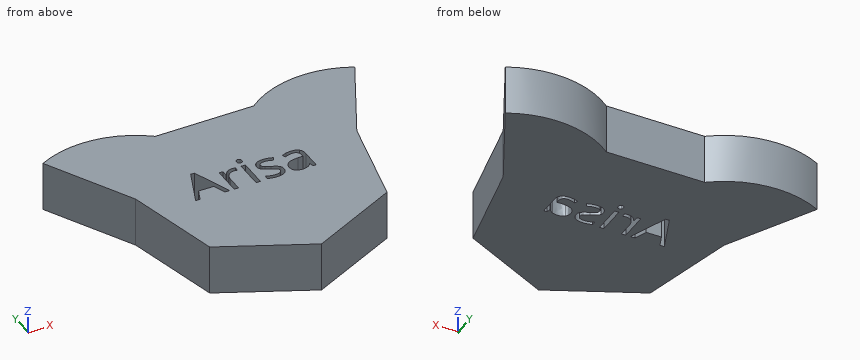
```python
from build123d import *

# Parameters (mm, degrees)
F0_W       = 2.2281454939
F0_H       = 14.7040429991
F1_DEPTH   = 25.4
F1_FACE_W  = 50.8
F1_FACE_H  = 25.4
F2_ANGLE   = 66
F1_FACE1_W = 50.8
F1_FACE1_H = 25.4
F3_ANGLE   = 66


with BuildPart() as f1:
    # F0 (on Top) → F1 (new body)
    with BuildSketch(Plane.XY):
        Polygon((-26.2134087423, 52.3441413045), (-57.2680906174, 12.1415700729), (-45.1987322015, -37.2038510665), (0.9061934483, -58.5340135326), (46.3287369485, -35.7868699324), (56.8647965925, 13.9085166461), (24.5805045719, 53.130506508), align=None)
        Polygon((-16.3552618695, -1.5368833827), (-18.7164950518, -1.5368833827), (-21.1592981077, 4.7010653699), (-29.0200580293, 4.7010653699), (-31.4328090265, -1.5368833827), (-33.742524394, -1.5368833827), (-25.9890932534, 18.1600945092), (-24.0700546489, 18.1600945092), align=None, mode=Mode.SUBTRACT)
        with BuildLine():
            add(Edge.make_bspline(
                [(-9.8210856812, 12.6584211944), (-8.6662279975, 13.4376281445), (-7.283833298, 13.4376281445)],
                knots=[0, 0, 0, 1, 1, 1], degree=2))
            add(Edge.make_bspline(
                [(-7.283833298, 13.4376281445), (-6.3049948152, 13.4376281445), (-5.5279344406, 13.2744883974)],
                knots=[0, 0, 0, 1, 1, 1], degree=2))
            Line((-5.5279344406, 13.2744883974), (-5.8370413299, 11.2094826507))
            add(Edge.make_bspline(
                [(-5.8370413299, 11.2094826507), (-6.747189393, 11.411260759), (-7.4469730452, 11.411260759)],
                knots=[0, 0, 0, 1, 1, 1], degree=2))
            add(Edge.make_bspline(
                [(-7.4469730452, 11.411260759), (-9.2329239613, 11.411260759), (-10.4994035773, 9.9623222153)],
                knots=[0, 0, 0, 1, 1, 1], degree=2))
            add(Edge.make_bspline(
                [(-10.4994035773, 9.9623222153), (-11.7658831932, 8.5133836715), (-11.7658831932, 6.3539285975)],
                knots=[0, 0, 0, 1, 1, 1], degree=2))
            Line((-11.7658831932, 6.3539285975), (-11.7658831932, -1.5368833827))
            Line((-11.7658831932, -1.5368833827), (-13.9940286871, -1.5368833827))
            Line((-13.9940286871, -1.5368833827), (-13.9940286871, 13.1671596164))
            Line((-13.9940286871, 13.1671596164), (-12.1565599561, 13.1671596164))
            Line((-12.1565599561, 13.1671596164), (-11.8989708817, 10.4453017298))
            Line((-11.8989708817, 10.4453017298), (-11.7916421007, 10.4453017298))
            add(Edge.make_bspline(
                [(-11.7916421007, 10.4453017298), (-10.975943365, 11.8792142442), (-9.8210856812, 12.6584211944)],
                knots=[0, 0, 0, 1, 1, 1], degree=2))
        make_face(mode=Mode.SUBTRACT)
        with Locations((-1.6619517484, 5.8151381168)):
            Rectangle(F0_W, F0_H, mode=Mode.SUBTRACT)
        with BuildLine():
            add(Edge.make_bspline(
                [(-2.5892724164, 16.0306914939), (-2.96492315, 16.3999025006), (-2.96492315, 17.1512039677)],
                knots=[0, 0, 0, 1, 1, 1], degree=2))
            add(Edge.make_bspline(
                [(-2.96492315, 17.1512039677), (-2.96492315, 17.9153848885), (-2.5892724164, 18.2717164415)],
                knots=[0, 0, 0, 1, 1, 1], degree=2))
            add(Edge.make_bspline(
                [(-2.5892724164, 18.2717164415), (-2.2136216829, 18.6280479944), (-1.6469257191, 18.6280479944)],
                knots=[0, 0, 0, 1, 1, 1], degree=2))
            add(Edge.make_bspline(
                [(-1.6469257191, 18.6280479944), (-1.110281814, 18.6280479944), (-0.7217516267, 18.2652767146)],
                knots=[0, 0, 0, 1, 1, 1], degree=2))
            add(Edge.make_bspline(
                [(-0.7217516267, 18.2652767146), (-0.3332214395, 17.9025054348), (-0.3332214395, 17.1512039677)],
                knots=[0, 0, 0, 1, 1, 1], degree=2))
            add(Edge.make_bspline(
                [(-0.3332214395, 17.1512039677), (-0.3332214395, 16.3999025006), (-0.7217516267, 16.0306914939)],
                knots=[0, 0, 0, 1, 1, 1], degree=2))
            add(Edge.make_bspline(
                [(-0.7217516267, 16.0306914939), (-1.110281814, 15.6614804872), (-1.6469257191, 15.6614804872)],
                knots=[0, 0, 0, 1, 1, 1], degree=2))
            add(Edge.make_bspline(
                [(-1.6469257191, 15.6614804872), (-2.2136216829, 15.6614804872), (-2.5892724164, 16.0306914939)],
                knots=[0, 0, 0, 1, 1, 1], degree=2))
        make_face(mode=Mode.SUBTRACT)
        with BuildLine():
            add(Edge.make_bspline(
                [(12.7394240882, 4.9028434782), (13.6581584537, 3.936884449), (13.6581584537, 2.472919876)],
                knots=[0, 0, 0, 1, 1, 1], degree=2))
            add(Edge.make_bspline(
                [(13.6581584537, 2.472919876), (13.6581584537, 0.420793583), (12.129796612, -0.693279164)],
                knots=[0, 0, 0, 1, 1, 1], degree=2))
            add(Edge.make_bspline(
                [(12.129796612, -0.693279164), (10.6014347704, -1.8073519109), (7.8366453714, -1.8073519109)],
                knots=[0, 0, 0, 1, 1, 1], degree=2))
            add(Edge.make_bspline(
                [(7.8366453714, -1.8073519109), (4.9130093766, -1.8073519109), (3.2773187539, -0.8800312429)],
                knots=[0, 0, 0, 1, 1, 1], degree=2))
            Line((3.2773187539, -0.8800312429), (3.2773187539, 1.1849745038))
            add(Edge.make_bspline(
                [(3.2773187539, 1.1849745038), (4.3377271103, 0.6483305987), (5.5505423358, 0.341370285)],
                knots=[0, 0, 0, 1, 1, 1], degree=2))
            add(Edge.make_bspline(
                [(5.5505423358, 0.341370285), (6.7633575613, 0.0344099713), (7.8924563376, 0.0344099713)],
                knots=[0, 0, 0, 1, 1, 1], degree=2))
            add(Edge.make_bspline(
                [(7.8924563376, 0.0344099713), (9.6354757412, 0.0344099713), (10.5735292873, 0.590373057)],
                knots=[0, 0, 0, 1, 1, 1], degree=2))
            add(Edge.make_bspline(
                [(10.5735292873, 0.590373057), (11.5115828334, 1.1463361426), (11.5115828334, 2.2883143727)],
                knots=[0, 0, 0, 1, 1, 1], degree=2))
            add(Edge.make_bspline(
                [(11.5115828334, 2.2883143727), (11.5115828334, 3.1469446208), (10.7688676688, 3.7565720969)],
                knots=[0, 0, 0, 1, 1, 1], degree=2))
            add(Edge.make_bspline(
                [(10.7688676688, 3.7565720969), (10.0261525041, 4.3661995731), (7.8624042789, 5.1990709138)],
                knots=[0, 0, 0, 1, 1, 1], degree=2))
            add(Edge.make_bspline(
                [(7.8624042789, 5.1990709138), (5.8102779859, 5.9632518346), (4.9452080109, 6.5342409496)],
                knots=[0, 0, 0, 1, 1, 1], degree=2))
            add(Edge.make_bspline(
                [(4.9452080109, 6.5342409496), (4.0801380359, 7.1052300646), (3.6572626387, 7.8286260487)],
                knots=[0, 0, 0, 1, 1, 1], degree=2))
            add(Edge.make_bspline(
                [(3.6572626387, 7.8286260487), (3.2343872415, 8.5520220327), (3.2343872415, 9.556619423)],
                knots=[0, 0, 0, 1, 1, 1], degree=2))
            add(Edge.make_bspline(
                [(3.2343872415, 9.556619423), (3.2343872415, 11.3554497928), (4.6983518145, 12.3965389687)],
                knots=[0, 0, 0, 1, 1, 1], degree=2))
            add(Edge.make_bspline(
                [(4.6983518145, 12.3965389687), (6.1623163876, 13.4376281445), (8.7081550733, 13.4376281445)],
                knots=[0, 0, 0, 1, 1, 1], degree=2))
            add(Edge.make_bspline(
                [(8.7081550733, 13.4376281445), (11.0822677093, 13.4376281445), (13.3533447156, 12.4716691154)],
                knots=[0, 0, 0, 1, 1, 1], degree=2))
            Line((13.3533447156, 12.4716691154), (12.5591117361, 10.6599592919))
            add(Edge.make_bspline(
                [(12.5591117361, 10.6599592919), (10.3481388472, 11.5701073549), (8.5493084774, 11.5701073549)],
                knots=[0, 0, 0, 1, 1, 1], degree=2))
            add(Edge.make_bspline(
                [(8.5493084774, 11.5701073549), (6.9651356696, 11.5701073549), (6.160169812, 11.0742483866)],
                knots=[0, 0, 0, 1, 1, 1], degree=2))
            add(Edge.make_bspline(
                [(6.160169812, 11.0742483866), (5.3552039544, 10.5783894183), (5.3552039544, 9.7068797164)],
                knots=[0, 0, 0, 1, 1, 1], degree=2))
            add(Edge.make_bspline(
                [(5.3552039544, 9.7068797164), (5.3552039544, 9.1144248452), (5.6578711168, 8.7001357505)],
                knots=[0, 0, 0, 1, 1, 1], degree=2))
            add(Edge.make_bspline(
                [(5.6578711168, 8.7001357505), (5.9605382793, 8.2858466558), (6.6302698728, 7.9101959222)],
                knots=[0, 0, 0, 1, 1, 1], degree=2))
            add(Edge.make_bspline(
                [(6.6302698728, 7.9101959222), (7.3000014664, 7.5345451887), (9.2061606172, 6.8218820827)],
                knots=[0, 0, 0, 1, 1, 1], degree=2))
            add(Edge.make_bspline(
                [(9.2061606172, 6.8218820827), (11.8206897227, 5.8688025073), (12.7394240882, 4.9028434782)],
                knots=[0, 0, 0, 1, 1, 1], degree=2))
        make_face(mode=Mode.SUBTRACT)
        with BuildLine():
            Line((27.9758178412, -1.5368833827), (26.3229546135, -1.5368833827))
            Line((26.3229546135, -1.5368833827), (25.8807600358, 0.5581744227))
            Line((25.8807600358, 0.5581744227), (25.7734312547, 0.5581744227))
            add(Edge.make_bspline(
                [(25.7734312547, 0.5581744227), (24.6743845371, -0.8242202768), (23.5817775464, -1.3157860938)],
                knots=[0, 0, 0, 1, 1, 1], degree=2))
            add(Edge.make_bspline(
                [(23.5817775464, -1.3157860938), (22.4891705557, -1.8073519109), (20.8491867817, -1.8073519109)],
                knots=[0, 0, 0, 1, 1, 1], degree=2))
            add(Edge.make_bspline(
                [(20.8491867817, -1.8073519109), (18.6639728003, -1.8073519109), (17.4232520917, -0.6782531346)],
                knots=[0, 0, 0, 1, 1, 1], degree=2))
            add(Edge.make_bspline(
                [(17.4232520917, -0.6782531346), (16.1825313832, 0.4508456417), (16.1825313832, 2.5287308421)],
                knots=[0, 0, 0, 1, 1, 1], degree=2))
            add(Edge.make_bspline(
                [(16.1825313832, 2.5287308421), (16.1825313832, 6.9807286786), (23.3048692914, 7.1953862407)],
                knots=[0, 0, 0, 1, 1, 1], degree=2))
            Line((23.3048692914, 7.1953862407), (25.7991901622, 7.2769561142))
            Line((25.7991901622, 7.2769561142), (25.7991901622, 8.1913973285))
            add(Edge.make_bspline(
                [(25.7991901622, 8.1913973285), (25.7991901622, 9.9215372785), (25.0564749976, 10.7458223167)],
                knots=[0, 0, 0, 1, 1, 1], degree=2))
            add(Edge.make_bspline(
                [(25.0564749976, 10.7458223167), (24.3137598329, 11.5701073549), (22.673776059, 11.5701073549)],
                knots=[0, 0, 0, 1, 1, 1], degree=2))
            add(Edge.make_bspline(
                [(22.673776059, 11.5701073549), (20.836307328, 11.5701073549), (18.5180056581, 10.4453017298)],
                knots=[0, 0, 0, 1, 1, 1], degree=2))
            Line((18.5180056581, 10.4453017298), (17.8311014596, 12.1496827724))
            add(Edge.make_bspline(
                [(17.8311014596, 12.1496827724), (18.9172687235, 12.7378444923), (20.2116538225, 13.0727102891)],
                knots=[0, 0, 0, 1, 1, 1], degree=2))
            add(Edge.make_bspline(
                [(20.2116538225, 13.0727102891), (21.5060389216, 13.4075760859), (22.8111568987, 13.4075760859)],
                knots=[0, 0, 0, 1, 1, 1], degree=2))
            add(Edge.make_bspline(
                [(22.8111568987, 13.4075760859), (25.438565458, 13.4075760859), (26.7071916496, 12.241985524)],
                knots=[0, 0, 0, 1, 1, 1], degree=2))
            add(Edge.make_bspline(
                [(26.7071916496, 12.241985524), (27.9758178412, 11.0763949622), (27.9758178412, 8.5005042178)],
                knots=[0, 0, 0, 1, 1, 1], degree=2))
            Line((27.9758178412, 8.5005042178), (27.9758178412, -1.5368833827))
        make_face(mode=Mode.SUBTRACT)
    extrude(amount=F1_DEPTH)

    # F1_face (on face) → F2 (revolve)
    with BuildSketch(Plane(origin=(40.7226505822, 33.519511577, 12.7), x_dir=(-0.6355175595, 0.7720864146, 0), z_dir=(0.7720864146, 0.6355175595, 0))):
        Rectangle(F1_FACE_W, F1_FACE_H)
    revolve(axis=Axis((56.8647965925, 13.9085166461, 12.7), (0, 0, -1)), revolution_arc=F2_ANGLE)

    # F1_face1 (on face) → F3 (revolve)
    with BuildSketch(Plane(origin=(-41.7407496799, 32.2428556887, 12.7), x_dir=(-0.6113126353, -0.7913891975, 0), z_dir=(-0.7913891975, 0.6113126353, 0))):
        Rectangle(F1_FACE1_W, F1_FACE1_H)
    revolve(axis=Axis((-57.2680906174, 12.1415700729, 12.7), (0, 0, 1)), revolution_arc=F3_ANGLE)


solid = f1.part
```
Here's how the part is built. I have some questions about the finished solid (model axes, mm). Coordinates: 2 decimals unless noted, no trailing zeros. Loops run counter-clockwise (first coordinate to the right, second up) from the corner with the lowest first, then second, coordinate; pieces in that order, holes last. Notation, with made-up numbers: (-23, 47) -> (25, 47) arc R19 cw to (25, 51) -> close; hole circle Ø7 at (34, 51.5). An arc over 180 degrees is marked (long way). Return JSON: item names as keys, results as strings.
1) If we section it at B-B, the plane y = -5.5: Write out the boundary of the cut face in (x, z).
Results below:
{"outline": "(-52.95, 0) -> (52.75, 0) -> (52.75, 25.4) -> (-52.95, 25.4) -> close"}
2) If we section it at A-A, the plane z = 20.5: Count the separate pieces of the cut face and the enclosed holes in it, then the cut area to 3 significant figures.
Results below:
{"separate pieces": "1", "enclosed holes": "6", "area": "12,000 mm²"}
3) I need wall thicknesses on line 1 (X direction, y = 16, z = 20.5); line 2 (Y direction, x = 24, z = 8); line 3 (Y direction, x = 22, z = 2.25). Which ranges of each line are inside material? Lowest first, please. Write a range as from..to.
Results below:
{"line 1": "-59.35..-26.84, -23.22..-2.56, -0.76..57.91", "line 2": "-46.97..-1.1, 7.22..11.39, 13.34..53.12", "line 3": "-47.97..-1.74, 7.11..11.53, 13.38..53.09"}
4) If we section it at C-C, the plane x = 52.5: Write out the boundary of the cut face in (y, z).
Results below:
{"outline": "(-6.68, 0) -> (64.52, 0) -> (64.52, 25.4) -> (-6.68, 25.4) -> close"}
5) Will these pins go through, and if not, where does the flat tip stop? pin 1 (0.5 mm diameter, centred on x = 26.5, z = 17.5, fed in from +Y); pin 2 (5 mm diameter, centred on x = 1, z = 12.5, fed in from +Y); pin 3 (2 mm diameter, centred on x = -13, z = 8.5, fed in from -Y).
Results below:
{"pin 1": "y = 54.82", "pin 2": "y = 52.8", "pin 3": "y = -52.56"}
